Input: dimensioned drawing with shaded views. Units: mm. Origin: part minimum x, y, z. A direction names the side the tool comes from. Round coordinates to 2 decimals unless told otherwise and drop trailing zeros. Order: outer loops, then holes, each group sorted by start corner. A loop starts at its lowest first (then second) coordinate and runs counter-clockwise, first axis right, second up.
Item 1: Cut plane A-A on y = 3. Output: boundary loops of the cut face in (x, z).
Item 2: Reachability of the marked faces 4 and 5 from +Z, -Z, +X, -X, +Y, -Y: full face, straight path, thin tool, end or side. Return the list, or none.
Item 3: Cut plane D-D on x = 1. Output: boundary loops of the cut face in (y, z), then the cut area to 3 significant figures.
Item 4: Cut plane C-C on x = 3.2. Output: boundary loops of the cut face in (y, z).
Item 5: Mould query, pull axis Y, two halves, no side actions, for the marked faces 1, 2 and 3. Classes: released by +Y, released by -Y, zero draft, split by the parting line, or undercut.
Item 6: Cut plane B-B on z = 1.85. Output: boundary loops of the cut face in (x, y).
Item 7: First-contact query: pin 1 (0.9 mm diameter, centred on y = 2.5, z = 2.5, fed in from +X); pin 2 (0.8 mm diameter, centred on y = 5, z = 0.5, fed in from -X); pin 3 (3 mm diameter, centred on x = 4, y = 2, fed in from -Z); pin 4 (0.9 mm diameter, centred on y = 3, z = 2.5, fed in from -X). Flat tips, straight axial feed; report the tip coordinate or a pass-through.
Item 8: Line query: L1, parallel to Z at x = 5.5, y = 2; L2, parallel to Z at x = 2, y = 2.1; L3, parallel to X at y = 4.8, z = 3.2. Output: solid intervals per line, ascending.
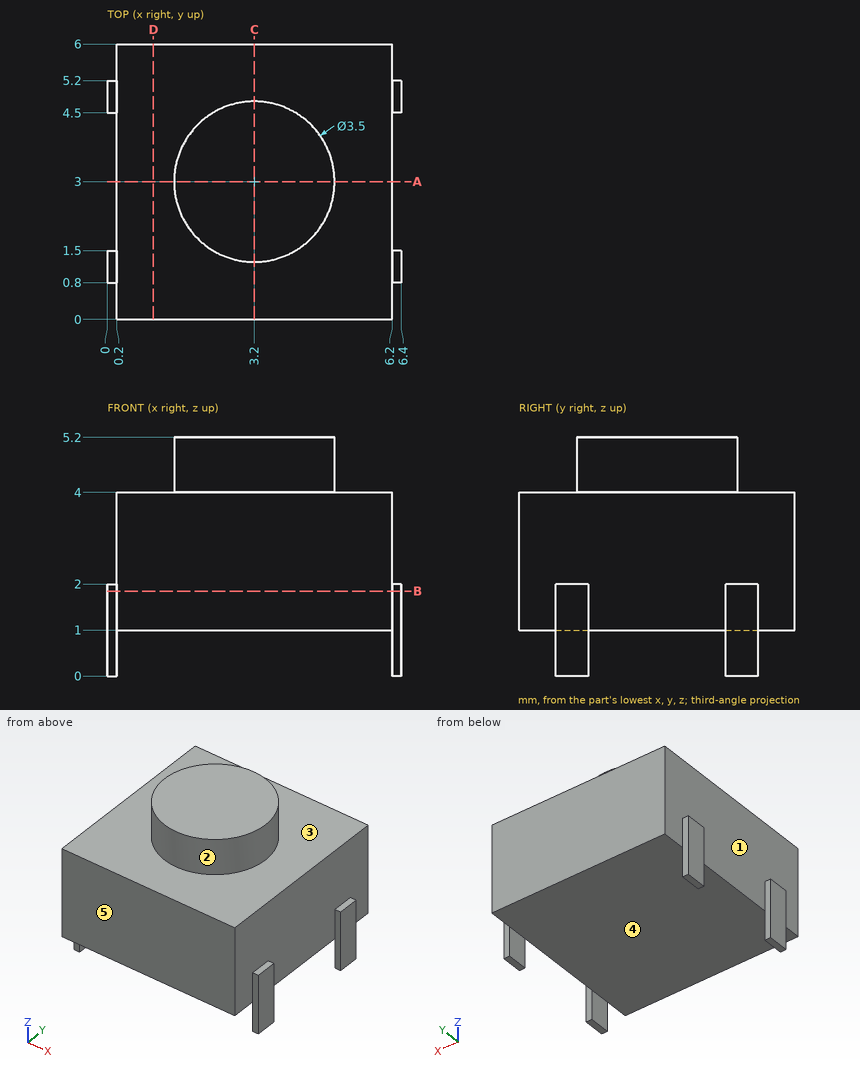
From the geometry:
1. outline: (0.2, 1) - (6.2, 1) - (6.2, 4) - (4.95, 4) - (4.95, 5.2) - (1.45, 5.2) - (1.45, 4) - (0.2, 4) - close
2. face 4: -Z, +Y, -Y
2. face 5: +Z, -Z, +X, -X, -Y
3. outline: (0, 1) - (6, 1) - (6, 4) - (0, 4) - close
3. area: 18.0 mm2
4. outline: (0, 1) - (6, 1) - (6, 4) - (4.75, 4) - (4.75, 5.2) - (1.25, 5.2) - (1.25, 4) - (0, 4) - close
5. face 1: undercut
5. face 2: split by the parting line
5. face 3: zero draft
6. outline: (0, 0.8) - (0.2, 0.8) - (0.2, 0) - (6.2, 0) - (6.2, 0.8) - (6.4, 0.8) - (6.4, 1.5) - (6.2, 1.5) - (6.2, 4.5) - (6.4, 4.5) - (6.4, 5.2) - (6.2, 5.2) - (6.2, 6) - (0.2, 6) - (0.2, 5.2) - (0, 5.2) - (0, 4.5) - (0.2, 4.5) - (0.2, 1.5) - (0, 1.5) - close
7. pin 1: stops at x = 6.2
7. pin 2: stops at x = 0
7. pin 3: stops at z = 1
7. pin 4: stops at x = 0.2
8. L1: z = 1 to 4
8. L2: z = 1 to 5.2
8. L3: x = 0.2 to 6.2
